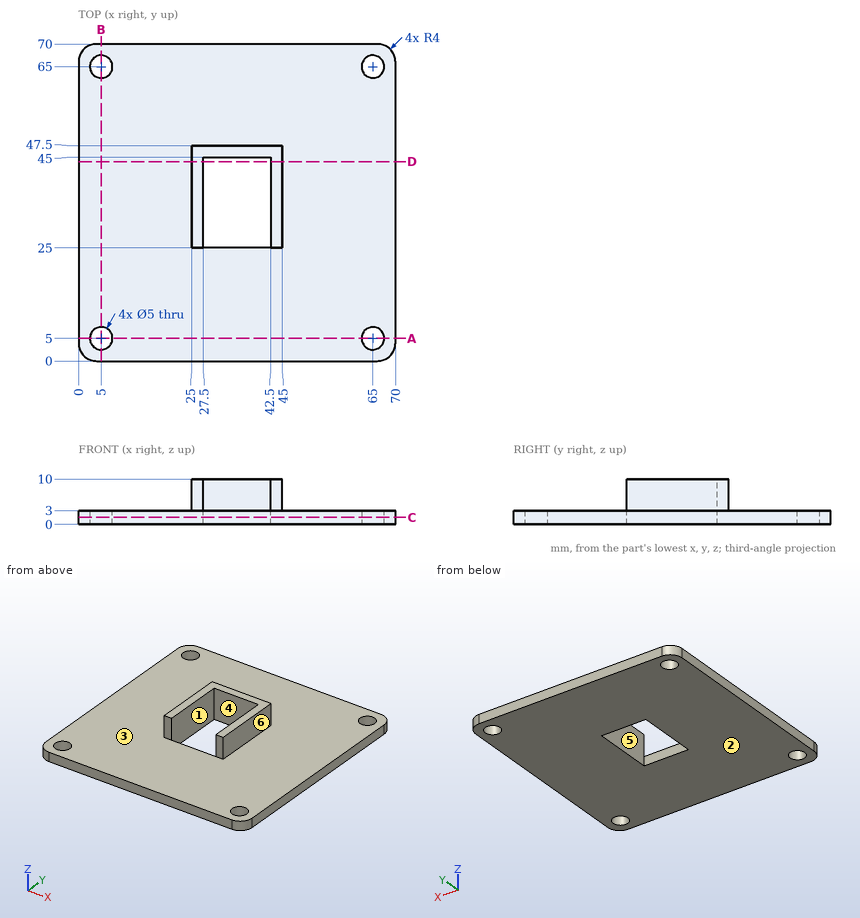
Can you work these out from the drawing? Everything is in mm from the part's minimum corner. A direction names the side the tool comes from. Coordinates: 2 decimals unless noted, no trailing zeros. Loops run counter-clockwise (first coordinate to the right, second up) from the corner with the lowest first, then second, coordinate; pieces in that order, holes last.
1. Imagine slicing it at A-A, the plane y = 5. Please give me the cut outline in (x, z).
2. Imagine slicing it at D-D, the plane y = 44. Please give me the cut outline in (x, z).
3. If we mould it in two halves opening along X, with no side actions, what happens to the marked faces 3, 4, 5 and 6? For each: pulls with the +X half, pulls with the -X half, needs draft (parallel to the pull), parting line crosses it, or undercut.
4. I need wall thicknesses on L1, parallel to Y at x = 5, z = 2.2; L2, parallel to X at y = 41.5, z = 0.5; L3, parallel to X at y = 44, z = 7.25. Which ranges of each line are inside material? Lowest first, please.
5. For the marked faces 1 and 2, which set-ups out of +Z, -Z, +X, -X, +Y, -Y let a thin tool reach every point of the face, with its end or its side?
6. Imagine slicing it at C-C, the plane z = 1.5. Please give me the cut outline in (x, y).
7. For P1, Ø3, axis at y = 33, z = 7, coming from the -X side; P2, Ø6.5, axis at x = 5, y = 5, coming from the +Z side; P3, Ø1.2, axis at x = 44.5, z = 8, coming from the -Y side, each with a flat end and sliding along its axis, tell me the tip position at first contact or that it passes through.
Taken from the geometry:
1. outline: (0, 0) - (2.5, 0) - (2.5, 3) - (0, 3) - close; (7.5, 0) - (62.5, 0) - (62.5, 3) - (7.5, 3) - close; (67.5, 0) - (70, 0) - (70, 3) - (67.5, 3) - close
2. outline: (0, 0) - (27.5, 0) - (27.5, 10) - (25, 10) - (25, 3) - (0, 3) - close; (42.5, 0) - (70, 0) - (70, 3) - (45, 3) - (45, 10) - (42.5, 10) - close
3. face 3: needs draft
3. face 4: undercut
3. face 5: undercut
3. face 6: pulls with the +X half
4. L1: y = 0 to 2.5, 7.5 to 62.5, 67.5 to 70
4. L2: x = 0 to 27.5, 42.5 to 70
4. L3: x = 25 to 27.5, 42.5 to 45
5. face 1: +Z, -Z
5. face 2: -Z, +X, -X, +Y, -Y
6. outline: (0, 4) arc R4 ccw to (4, 0) - (66, 0) arc R4 ccw to (70, 4) - (70, 66) arc R4 ccw to (66, 70) - (4, 70) arc R4 ccw to (0, 66) - close; hole circle Ø5 at (5, 5); hole circle Ø5 at (5, 65); hole (27.5, 25) - (42.5, 25) - (42.5, 45) - (27.5, 45) - close; hole circle Ø5 at (65, 5); hole circle Ø5 at (65, 65)
7. P1: stops at x = 25
7. P2: stops at z = 3
7. P3: stops at y = 25
